from build123d import *

# Parameters (mm, degrees)
SKETCH1_R               = 42.5
BOSS_EXTRUDE1_DEPTH     = 5
SKETCH2_R               = 42.5
SKETCH2_R_2             = 40
BOSS_EXTRUDE2_DEPTH     = 30
SKETCH3_R               = 2
BOSS_EXTRUDE3_DEPTH     = 5
CUT_EXTRUDE1_DEPTH      = 70.552138838
CUT_EXTRUDE1_DEPTH_BACK = 70.552138838
SKETCH3_3_R             = 2
CUT_EXTRUDE4_REACH      = 71.552
CUT_EXTRUDE4_END_RADIUS = 42.5
SKETCH4_R               = 2.5
CUT_EXTRUDE8_START      = 50
SKETCH4_5_R             = 5
SKETCH4_5_R_2           = 2.5
CUT_EXTRUDE8_DEPTH      = 50


with BuildPart() as part:
    # Sketch1 → Boss-Extrude1 (new body)
    with BuildSketch(Plane(origin=(0, 0, 0), x_dir=(1, 0, 0), z_dir=(0, 1, 0))):
        with Locations(Location((0, 0, 0), (0, 0, 270))):
            Circle(SKETCH1_R)
    extrude(amount=BOSS_EXTRUDE1_DEPTH)

    # Sketch2 → Boss-Extrude2 (add)
    with BuildSketch(Plane(origin=(0, 5, 0), x_dir=(1, 0, 0), z_dir=(0, 1, 0))):
        with Locations(Location((0, 0, 0), (0, 0, 270))):
            Circle(SKETCH2_R)
        with Locations(Location((0, 0, 0), (0, 0, 270))):
            Circle(SKETCH2_R_2, mode=Mode.SUBTRACT)
    extrude(amount=BOSS_EXTRUDE2_DEPTH)

    # Sketch3 → Boss-Extrude3 (add)
    with BuildSketch(Plane.XZ):
        with BuildLine():
            ThreePointArc((-25.178047354, -16.486591759), (-14.183962111, -19.037364236), (-7.815144583, -9.719933589))
            ThreePointArc((-7.815144583, -9.719933589), (-12.938182194, 0.241771609), (-7.410610084, 9.984822024))
            ThreePointArc((-7.410610084, 9.984822024), (-14.893502945, 19.290955178), (-25.95577439, 14.793850517))
            add(Edge.make_bspline(
                [(-25.95577439, 14.793850517), (-26.206471304, 14.310519768), (-26.451758672, 13.821089407), (-26.688052402, 13.325870914)],
                knots=[0, 0, 0, 0, 0.050650552, 0.050650552, 0.050650552, 0.050650552], degree=3))
            add(Edge.make_bspline(
                [(-26.688052402, 13.325870914), (-27.746594537, 11.107404767), (-28.624649084, 8.772780294), (-29, 6.35)],
                knots=[0.050650552, 0.050650552, 0.050650552, 0.050650552, 0.277553495, 0.277553495, 0.277553495, 0.277553495], degree=3))
            add(Edge.make_bspline(
                [(-29, 6.35), (-30.042272144, 0), (-29, -6.35)],
                knots=[0, 0, 0, 1, 1, 1], degree=2))
            add(Edge.make_bspline(
                [(-29, -6.35), (-28.699050384, -11.600454078), (-25.178047354, -16.486591759)],
                knots=[0.67268265, 0.67268265, 0.67268265, 1, 1, 1], degree=2))
        make_face()
        with Locations(Location((-24.5, 0, 0), (0, 0, 90))):
            Circle(SKETCH3_R, mode=Mode.SUBTRACT)
        with Locations(Location((-17.25, 0, 0), (0, 0, 90))):
            Circle(SKETCH3_R, mode=Mode.SUBTRACT)
    extrude(amount=BOSS_EXTRUDE3_DEPTH)

    # Sketch3_3 → Cut-Extrude1 (cut, two sides: drawn at the far end of the back side and taken through both)
    with BuildSketch(Plane.XZ.offset(-CUT_EXTRUDE1_DEPTH_BACK)):
        with Locations(Location((-17.25, 0, 0), (0, 0, 90))):
            Circle(SKETCH3_3_R)
        with Locations(Location((-24.5, 0, 0), (0, 0, 90))):
            Circle(SKETCH3_3_R)
    extrude(amount=CUT_EXTRUDE1_DEPTH + CUT_EXTRUDE1_DEPTH_BACK, mode=Mode.SUBTRACT)

    # Cut-Extrude4: up to this cylinder (the profile starts inside it)
    cut_extrude4_end = Plane(origin=(0, 15, 0), z_dir=(0, -1, 0)) * Cylinder(CUT_EXTRUDE4_END_RADIUS, 229.104, mode=Mode.PRIVATE)
    # Sketch4 → Cut-Extrude4 (cut, up to the surface)
    with BuildSketch(Plane(origin=(0, 0, 0), x_dir=(0, 0, -1), z_dir=(1, 0, 0)), mode=Mode.PRIVATE) as cut_extrude4_sk1:
        with Locations((0, 15)):
            Circle(SKETCH4_R)
    cut_extrude4_tool1 = extrude(cut_extrude4_sk1.sketch, amount=-CUT_EXTRUDE4_REACH, mode=Mode.PRIVATE) & cut_extrude4_end
    add(cut_extrude4_tool1.solids().sort_by_distance((0, 15, 0))[0], mode=Mode.SUBTRACT)

    # Sketch4_5 → Cut-Extrude8 (cut)
    # profile 1 of 2: a face of its own
    with BuildSketch(Plane(origin=(0, 0, 0), x_dir=(0, 0, -1), z_dir=(1, 0, 0)).offset(CUT_EXTRUDE8_START)):
        with Locations(Location((0, 15, 0), (0, 0, 180))):
            Circle(SKETCH4_5_R)
        with Locations((0, 15)):
            Circle(SKETCH4_5_R_2, mode=Mode.SUBTRACT)
    # profile 2 of 2: a face of its own
    with BuildSketch(Plane(origin=(0, 0, 0), x_dir=(0, 0, -1), z_dir=(1, 0, 0)).offset(CUT_EXTRUDE8_START)):
        with Locations((0, 15)):
            Circle(SKETCH4_5_R_2)
    extrude(amount=-CUT_EXTRUDE8_DEPTH, mode=Mode.SUBTRACT)


solid = part.part
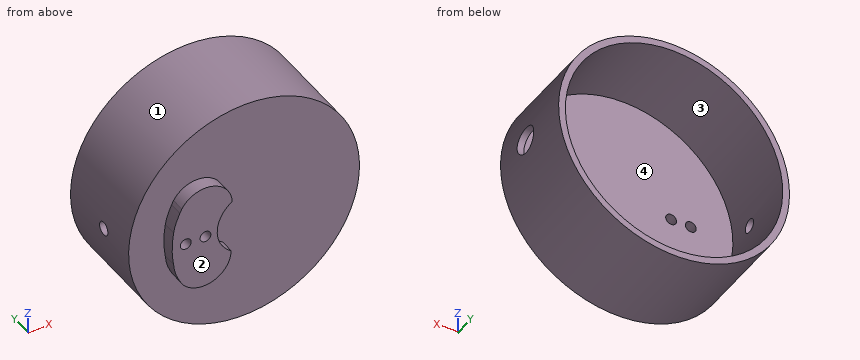
For this review, take the finished solid that the model builds, in its own axes (mm). Face numbers are marked on the shaded views. Give positions to 0.01 mm unless a question says otherwise; leave off trailing zeros. Loops run counter-clockwise (first coordinate to the right, second up) from the corner with the lowest first, then second, coordinate; pieces in that order, holes last. Notation, with made-up numbers: M 10,80.25 L 37,80.25 A18 ccw 37,94.25 Z; hole C 34.5,87.25 d5. An arc over 180 degrees is marked long. Answer as a JSON object with one key per item and string values. Group by question number.
Q1. Add section B-B on z = 0. Give the number of separate pieces and of enclosed holes in the cut face, and give its area (3 significant figures).
Q2. For probe 1 along X at (y, z) = (2, 0); probe 2 along X at (y, z) = (-1, 0); probe 3 along X at (y, z) = (26, 0), list the stretches that pass through material, from the lowest coordinate up. Write a range as [from, to].
Q3. Insertion check: P1, Ø10, axis at y = 19, z = -28.5, coming from the +X side; P2, Ø5, axis at x = 13.5, y = 16, coming from the -Z side; P3, Ø3, axis at x = 11.5, z = -31.5, coming from the -Y side. Each pin has a flat end and moves straight along its axis. Give the tip position at first contact, or say it passes through.
Q4. Add section A-A on x = -17.25. Give the boundary of the cut face in (y, z).
Q5. Mouldability with a two-part tool opening along Z and no side actions: class the marked faces 1, 2, 3 and 4 as +Z half, -Z half, draft (parallel to the pull), parting line (faces both ways), or undercut.
Q6. Add section C-C on x = 0. Give the boundary of the cut face in (y, z), and give its area (3 significant figures).
Q7. Add section D-D on y = 23. Give the boundary of the cut face in (x, z), and give its area (3 significant figures).
Checked values:
{
 "1": {"separate pieces": "5", "enclosed holes": "0", "area": "540 mm²"},
 "2": {"probe 1": "[-42.5, -26.5], [-22.5, -19.25], [-15.25, 42.5]", "probe 2": "[-29.52, -26.5], [-22.5, -19.25], [-15.25, -12.94]", "probe 3": "[-42.5, -40], [40, 42.5]"},
 "3": {"P1": "x = 35.41", "P2": "z = -41.05", "P3": "y = 0"},
 "4": {"outline": "M -5,-19.7 L 0,-19.7 L 0,-38.84 L 35,-38.84 L 35,-36.09 L 5,-36.09 L 5,-2 L -5,-2 Z; M -5,2 L 5,2 L 5,36.09 L 35,36.09 L 35,38.84 L 0,38.84 L 0,19.61 L -5,19.61 Z"},
 "5": {"face 1": "parting line", "face 2": "draft", "face 3": "undercut", "face 4": "undercut"},
 "6": {"outline": "M 0,-42.5 L 35,-42.5 L 35,-40 L 5,-40 L 5,40 L 35,40 L 35,42.5 L 0,42.5 Z", "area": "575 mm²"},
 "7": {"outline": "C 0,0 d85; hole C 0,0 d80", "area": "648 mm²"}
}
